Source: CAD feature listing. Evaluate the final solid. Frame: model axes, mm. A direction names the side the tool comes from. Round coordinates to 2 decimals unless told otherwise and drop trailing zeros. Write each loop counter-clockwise with the first axis right and the second up, starting at its lowest first coordinate (ties: lowest second). Pieces come first, ordered by that corner, then holes.
from build123d import *

# Parameters (mm, degrees)
SKETCH1_R           = 25
SKETCH1_R_2         = 10
BOSS_EXTRUDE1_DEPTH = 80.5
SKETCH3_W           = 6
SKETCH3_H           = 2.8
CUT_EXTRUDE1_DEPTH  = 80.5


with BuildPart() as part:
    # Sketch1 → Boss-Extrude1 (new, symmetric)
    with BuildSketch(Plane(origin=(0, 0, 0), x_dir=(0, 0, -1), z_dir=(1, 0, 0))):
        Circle(SKETCH1_R)
        Circle(SKETCH1_R_2, mode=Mode.SUBTRACT)
    extrude(amount=BOSS_EXTRUDE1_DEPTH, both=True)

    # Sketch3 → Cut-Extrude1 (cut, symmetric)
    with BuildSketch(Plane(origin=(0, 0, 0), x_dir=(0, 0, -1), z_dir=(1, 0, 0))):
        with Locations((0, 10)):
            Rectangle(SKETCH3_W, SKETCH3_H)
    extrude(amount=CUT_EXTRUDE1_DEPTH, both=True, mode=Mode.SUBTRACT)


solid = part.part
1) Section query D-D on y = -20.5. Return the cut outline in (x, z).
Taken from the geometry:
outline: (-80.5, -14.31) - (80.5, -14.31) - (80.5, 14.31) - (-80.5, 14.31) - close
2) Section query B-B on x = -20.5. Return the cut outline in (y, z).
Taken from the geometry:
outline: circle Ø50 at (0, 0); hole (9.54, -3) - (11.4, -3) - (11.4, 3) - (9.54, 3) arc R10 ccw (long way) to start
3) Contact query for flat-ended pins moving along their axis: P1, Ø1.5, axis at x = 31, z = 12, coming from the -Y side; P2, Ø6, axis at x = 11.5, y = -19.5, coming from the +Z side; P3, Ø4, axis at x = 5.5, y = 10.5, coming from the -Z side. Output: stop coordinate, or through.
Taken from the geometry:
P1: stops at y = -22.33
P2: stops at z = 18.78
P3: stops at z = -23.51
4) Material intervals for line 1 (Y direction, x = 12, z = 0); line 2 (Z direction, x = -2, y = 1.5); line 3 (Y direction, x = -56.5, z = 1), sorted ascending.
Taken from the geometry:
line 1: y = -25 to -10, 11.4 to 25
line 2: z = -24.95 to -9.89, 9.89 to 24.95
line 3: y = -24.98 to -9.95, 11.4 to 24.98
5) Pull-direction query (Y, two-part tool) for faces 3 (the face through (1.127, 7.509, -23.846)), 4 (the face through (80.5, -11, 0)), 5 (the face through (-1, -10, 0)); classes: released by +Y, released by -Y, zero draft, split by the parting line, or undercut.
Taken from the geometry:
face 3: split by the parting line
face 4: zero draft
face 5: undercut
6) Section query A-A on y = 0. Return the cut outline in (x, z), then the cut area to 3 significant figures.
Taken from the geometry:
outline: (-80.5, -25) - (80.5, -25) - (80.5, -10) - (-80.5, -10) - close; (-80.5, 10) - (80.5, 10) - (80.5, 25) - (-80.5, 25) - close
area: 4,830 mm2
7) Section query C-C on z = 0. Return the cut outline in (x, y), then the cut area to 3 significant figures.
Taken from the geometry:
outline: (-80.5, -25) - (80.5, -25) - (80.5, -10) - (-80.5, -10) - close; (-80.5, 11.4) - (80.5, 11.4) - (80.5, 25) - (-80.5, 25) - close
area: 4,600 mm2
8) Reachability of faces 1 (the face through (1, 11.4, 0)), 2 (the face through (-80.5, -11, 0)) from +Z, -Z, +X, -X, +Y, -Y: full face, straight path, thin tool, end or side. Return the list, or none.
Taken from the geometry:
face 1: +X, -X
face 2: +Z, -Z, -X, +Y, -Y
